Read the model definition and answer for the solid it produces. Units are mm, in the model's axes. Face numbers are marked on the shaded views. A direction names the side the tool comes from. Coordinates: 2 decimals unless noted, no trailing zeros. Write each loop counter-clockwise with the first axis right and the second up, starting at its lowest first coordinate (ties: lowest second). Pieces come first, ordered by that corner, then holes.
Item 1: Each of these flat-tipped pins is pushed along its axis until it touches: P1, Ø4.5, axis at y = 0, z = 10, coming from the +X side; P2, Ø1.2, axis at y = 41, z = 13, coming from the -X side; P3, Ø3.5, axis at y = 0, z = 10, coming from the +X side; P4, Ø2, axis at x = -14, z = 7.5, coming from the -Y side. Where does it stop, or does it pass through?
Item 2: Straight lines are drawn through the part: probe 1 along Z at (x, y) = (179, -40); probe 2 along Y at (x, z) = (-1.4, 10); probe 3 along Y at (x, z) = (9.5, 7). For each, find the intervals that lie inside material, in ascending order.
Item 3: A tool of negligible diameter and unlimited length cuts with its end or side. For the marked faces 5 and 6, from which of +Z, -Z, +X, -X, +Y, -Y can it reach the whole face along a straight path? Write none if from no direction.
Item 4: Section C-C (z = 2.75) is taken. Give the vertices of the cut face in (x, y).
Item 5: Determine the mould class of the marked faces 1, 2, 3 and 4 for opening direction Y: released by +Y, released by -Y, zero draft, split by the parting line, or undercut.
Item 6: Section B-B (x = 66) is taken. Give the vertices of the cut face in (y, z), then the cut area to 3 significant figures.
Item 7: Section A-A (x = 179) is taken. Give the vertices of the cut face in (y, z).
Item 8: Section D-D (y = 4.5) is taken. Give the vertices of the cut face in (x, z), then the cut area to 3 significant figures.
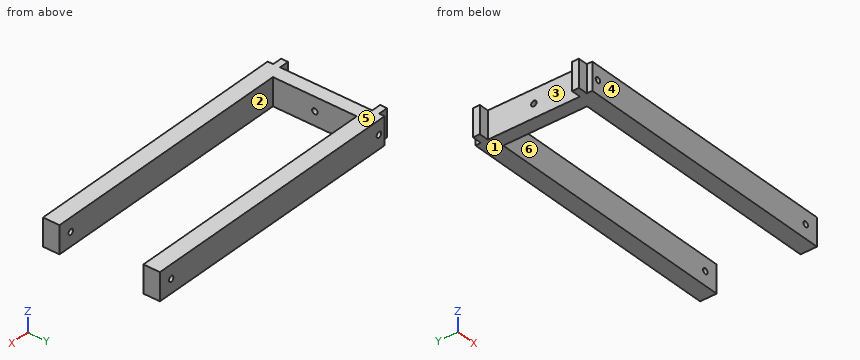
from build123d import *

# Parameters (mm, degrees)
PAD_DEPTH       = 20
SKETCH004_R     = 2
POCKET002_DEPTH = 199.001
SKETCH005_R     = 2
POCKET003_DEPTH = 85.001


with BuildPart() as part:
    # Sketch → Pad (new body)
    with BuildSketch(Plane.XY):
        Polygon((-10, -42.5), (189, -42.5), (189, -30.5), (0, -30.5), (0, 30.5), (189, 30.5), (189, 42.5), (-10, 42.5), (-10, 38.5), (-17, 38.5), (-17, 33.5), (-10, 33.5), (-10, -33.5), (-17, -33.5), (-17, -38.5), (-10, -38.5), align=None)
    extrude(amount=PAD_DEPTH)

    # Sketch004 → Pocket002 (cut, through all)
    with BuildSketch(Plane(origin=(-10, 0, 0), x_dir=(0, -1, 0), z_dir=(-1, 0, 0))):
        with Locations((0, 10)):
            Circle(SKETCH004_R)
    extrude(amount=-POCKET002_DEPTH, mode=Mode.SUBTRACT)

    # Sketch005 → Pocket003 (cut, through all)
    with BuildSketch(Plane.XZ.offset(42.5)):
        with Locations((-5, 10)):
            Circle(SKETCH005_R)
        with Locations((179, 10)):
            Circle(SKETCH005_R)
    extrude(amount=-POCKET003_DEPTH, mode=Mode.SUBTRACT)


solid = part.part
Established:
1. P1: stops at x = 0
1. P2: stops at x = -10
1. P3: passes through
1. P4: stops at y = -38.5
2. probe 1: z = 0 to 8, 12 to 20
2. probe 2: y = -42.5 to -2, 2 to 42.5
2. probe 3: y = -42.5 to -30.5, 30.5 to 42.5
3. face 5: +Z, +X, -X, +Y, -Y
3. face 6: +Z, -Z, +X
4. outline: (-17, -38.5) - (-10, -38.5) - (-10, -42.5) - (189, -42.5) - (189, -30.5) - (0, -30.5) - (0, 30.5) - (189, 30.5) - (189, 42.5) - (-10, 42.5) - (-10, 38.5) - (-17, 38.5) - (-17, 33.5) - (-10, 33.5) - (-10, -33.5) - (-17, -33.5) - close
5. face 1: zero draft
5. face 2: undercut
5. face 3: undercut
5. face 4: released by -Y
6. outline: (-42.5, 0) - (-30.5, 0) - (-30.5, 20) - (-42.5, 20) - close; (30.5, 0) - (42.5, 0) - (42.5, 20) - (30.5, 20) - close
6. area: 480 mm2
7. outline: (-42.5, 0) - (-30.5, 0) - (-30.5, 8) - (-42.5, 8) - close; (-42.5, 12) - (-30.5, 12) - (-30.5, 20) - (-42.5, 20) - close; (30.5, 0) - (42.5, 0) - (42.5, 8) - (30.5, 8) - close; (30.5, 12) - (42.5, 12) - (42.5, 20) - (30.5, 20) - close
8. outline: (-10, 0) - (0, 0) - (0, 20) - (-10, 20) - close; hole circle Ø4 at (-5, 10)
8. area: 187 mm2
